Could you check a few things on this model? Use its own coordinates, in mm. A direction names the side the tool comes from. Round coordinates to 2 decimals unless told otherwise and drop trailing zeros. Order: outer loops, then holes, each group sorted by start corner. A loop starts at its lowest first (then second) coordinate and runs counter-clockwise, first axis right, second up. Notation, with made-up numbers: (29.25, -7) - (79.25, -7) arc R18 cw to (79.25, 2) - close; hole circle Ø11 at (77, 60). An arc over 180 degrees is marked (long way). Use one line per item in the form item = value.
from build123d import *

# Parameters (mm, degrees)
F1_DEPTH = 31.75
F3_D     = 2.54


with BuildPart() as f1:
    # F0 (on Top) → F1 (new body)
    with BuildSketch(Plane.XY):
        Polygon((-7.939773, 39.316174), (-30.21069, 39.316174), (-41.346149, 20.028993), (-30.21069, 0.741813), (-7.939773, 0.741813), (3.195686, 20.028993), align=None)
        Polygon((-36.696177, 20.028993), (-27.885704, 35.28918), (-10.264759, 35.28918), (-1.454287, 20.028993), (-10.264759, 4.768807), (-27.885704, 4.768807), align=None, mode=Mode.SUBTRACT)
    extrude(amount=F1_DEPTH)

    # F3 (through all)
    with Locations(Plane.YZ):
        with Locations((10.597352, 25.751563), (31.580105, 25.751563), (31.580105, 10.279431), (10.597352, 10.279431)):
            Hole(F3_D / 2)


solid = f1.part
Item 1: For faces 1 (the face through (-35.7, 29.81, 15.65)), 2 (the face through (-32.23, 12.29, 15.65)), which set-ups out of +Z, -Z, +X, -X, +Y, -Y let a thin tool reach every point of the face, with its end or its side?
Found:
face_1 = +Z, -Z, -X, +Y
face_2 = +Z, -Z
Item 2: I need wall thicknesses on L1, parallel to Y at x = -11.5, z = 14; L2, parallel to Y at x = -31.5, z = 11; L3, parallel to X at y = 8.5, z = 15. Which ranges of each line are inside material? Lowest first, please.
Found:
L1 = 0.74 to 4.77, 35.29 to 39.32
L2 = 2.97 to 9.55, 29.03 to 30.53, 32.63 to 37.08
L3 = -34.69 to -30.04, -8.11 to -3.46
Item 3: Imagine slicing it at B-B on y = 10.5. Please give me the cut outline in (x, z), plus the area to 3 significant figures.
Found:
outline = (-35.84, 0) - (-31.19, 0) - (-31.19, 9.01) - (-35.84, 9.01) - close; (-35.84, 11.55) - (-31.19, 11.55) - (-31.19, 24.49) - (-35.84, 24.49) - close; (-35.84, 27.02) - (-31.19, 27.02) - (-31.19, 31.75) - (-35.84, 31.75) - close; (-6.96, 0) - (-2.31, 0) - (-2.31, 9.01) - (-6.96, 9.01) - close; (-6.96, 11.55) - (-2.31, 11.55) - (-2.31, 24.49) - (-6.96, 24.49) - close; (-6.96, 27.02) - (-2.31, 27.02) - (-2.31, 31.75) - (-6.96, 31.75) - close
area = 248 mm2
Item 4: Will these pins go through, and if not, where does the flat tip stop? P1, Ø2, axis at y = 31.58, z = 25.75, coming from the +X side; P2, Ø6, axis at y = 8, z = 4, coming from the -X side; P3, Ø3.5, axis at y = 31.58, z = 10.28, coming from the +X side; P4, Ø4, axis at x = -35, z = 20.5, coming from the +Y side.
Found:
P1 = through
P2 = -36.13
P3 = -2.46
P4 = 34.48
Item 5: Imagine slicing it at D-D on y = 26. Please give me the cut outline in (x, z).
Found:
outline = (-37.9, 0) - (-33.25, 0) - (-33.25, 31.75) - (-37.9, 31.75) - close; (-4.9, 0) - (-0.25, 0) - (-0.25, 31.75) - (-4.9, 31.75) - close
Item 6: If we mould it in two halves opening along X, with no side actions, what happens to faces 3 (the face through (-19, 4.769, 16)), 4 (the face through (-35.856, 10.52, 15.653)), 5 (the face through (-19, 39.316, 16))? For each: released by +X, released by -X, zero draft, split by the parting line, or undercut.
Found:
face_3 = undercut
face_4 = released by -X
face_5 = zero draft
Item 7: Imagine slicing it at A-A on x = -27. Please give me the cut outline in (y, z), plus the area to 3 significant figures.
Found:
outline = (0.74, 0) - (4.77, 0) - (4.77, 31.75) - (0.74, 31.75) - close; (35.29, 0) - (39.32, 0) - (39.32, 31.75) - (35.29, 31.75) - close
area = 256 mm2
Item 8: Imagine slicing it at C-C on z = 8. Please give me the cut outline in (x, y), plus the area to 3 significant figures.
Found:
outline = (-41.35, 20.03) - (-30.21, 0.74) - (-7.94, 0.74) - (3.2, 20.03) - (-7.94, 39.32) - (-30.21, 39.32) - close; hole (-36.7, 20.03) - (-27.89, 4.77) - (-10.26, 4.77) - (-1.45, 20.03) - (-10.26, 35.29) - (-27.89, 35.29) - close
area = 482 mm2
